The model under review builds one solid part; all positions refer to its coordinate system, in mm. A direction names the side the tool comes from. Round coordinates to 2 decimals unless told otherwise and drop trailing zeros. Loops run counter-clockwise (first coordinate to the right, second up) from the corner with the lowest first, then second, coordinate; pieces in that order, holes last. Notation, with made-up numbers: (8, -32) -> (65, -32) arc R24 ccw to (65, -20) -> close; hole circle Ø9 at (-5.75, -0.75). An arc over 180 degrees is marked (long way). Use a Markdown table: item, result. Add a question column.
1) Consider section C-C on z = 8. Give the boundary of the cut face in (x, y), plus the area to 3 significant figures.
2) Mouldability with a two-part tool opening along X and no side actions: class faces 1 (the cylindrical face through (2.285, 3.584, 14.521)), 2 (the flat face through (13.192, 4.676, 7.888)), 3 (the cylindrical face through (2.285, 3.584, 1.521)), 4 (the flat face through (6, 0, 16)) as released by +X, released by -X, zero draft, split by the parting line, or undercut.
3) For faces 5 (the flat face through (18, 2, 6)), 6 (the flat face through (5, 0, 3)), list the 3-axis set-ups (+Z, -Z, +X, -X, +Y, -Y) from which the entire face can be reached by the end or side of a thin tool; tool diameter is ignored.
4) Consider section D-D on x = 7.5. Give the boundary of the cut face in (y, z).
5) Insertion check: pin 1 (5 mm diameter, centred on x = 2, z = 12, fed in from -Y); pin 2 (1 mm diameter, centred on x = 12, z = 9.5, fed in from +Y); pin 3 (3 mm diameter, centred on x = 14.5, z = 2, fed in from +Y); pin 4 (1.5 mm diameter, centred on x = -3.5, z = 14, fed in from -Y). Each pin has a flat end and moves straight along its axis. Give the tip position at first contact, or say it passes through.
6) Consider section A-A on y = 0. Give the boundary of the cut face in (x, z).
7) Wall thickness on probe 1 along Z at (x, y) = (-4, 4); probe 2 along Y at (x, z) = (0, 13.95); probe 3 along Z at (x, y) = (16.25, 0): over which ranges is each line inside the solid? List them lowest first.
Autodesk Inventor part; units mm, degrees
ref_plane "Work Plane1" through (0, 6.5, 0) normal (0, 1, 0) x (-1, 0, 0)
ref_plane "YZ Plane" through (0, 0, 0) normal (1, 0, 0) x (0, 1, 0)
ref_plane "XY Plane" through (0, 0, 0) normal (0, 0, 1) x (1, 0, 0)
sketch "Sketch1" plane through (0, 0, 0) normal (0, 0, 1) x (1, 0, 0)
  arc A0 (0.2442, 6.4954) -> (0.2442, -6.4954) centre (0, 0) ccw
  line L0 (18, 4) -> (18, -4)
  line L1 (18, 4) -> (0.2442, 6.4954)
  line L2 (0.2442, -6.4954) -> (18, -4)
  point P0 (18, 0)
  dimension "d0" = 13
  dimension "d1" = 8
  dimension "d2" = 18
  dimension "d3" = 82
  dimension "d4" = 82
extrude "Extrusion1" add sketch "Sketch1" along normal blind 16
sketch "Sketch2" plane through (0, 0, 16) normal (0, 0, 1) x (1, 0, 0)
  arc A0 (0.2442, 6.4954) -> (0.2442, -6.4954) centre (0, 0) ccw
  circle A1 centre (0, 0) radius 4.25
  dimension "d7" = 8.5
extrude "Extrusion2" cut sketch "Sketch2" against normal through all
ref_plane "Work Plane1" through (0, 6.5, 0) normal (0, 1, 0) x (-1, 0, 0)
sketch "Sketch3" plane through (0, 6.5, 0) normal (0, 1, 0) x (-1, 0, 0)
  line L0 (6.5, 0) -> (6.5, 16)
  line L1 (6.5, 13) -> (-12, 13)
  line L2 (-12, 13) -> (-12, 3)
  line L3 (-12, 3) -> (6.5, 3)
  line L4 (6.5, 3) -> (6.5, 13)
  line L5 (-18, 0) -> (-18, 16)
  line L6 (6.5, 0) -> (-0.2442, 0)
  line L7 (6.5, 16) -> (-0.2442, 16)
  point P0 (0, 0)
  point P1 (6.5, 3)
  dimension "d11" = 6
  dimension "d12" = 3
  dimension "d13" = 3
extrude "Extrusion3" cut sketch "Sketch3" against normal through all
sketch "Sketch4" plane through (12, -4.8432, 3) normal (-1, 0, 0) x (0, 0, 1)
  line L0 (10, 9.6865) -> (10, 0)
  circle A0 centre (5, 4.8432) radius 2.5
  line L1 (-3, 8.8432) -> (13, 8.8432)
  point P0 (-3, 4.8432)
  dimension "d16" = 5
  dimension "d17" = 4
  dimension "d18" = 5
hole "Hole1" at (12, 0, 8) direction (1, 0, 0) diameter 4.917 depth 6
properties part number "16C - Con Head Crosshead" material "Steel AISI 1020 107 HR"
Result set:
| question | item | result |
|---|---|---|
| 1 | outline | (12, -4.84) -> (18, -4) -> (18, -2.46) -> (12, -2.46) -> close; (12, 2.46) -> (18, 2.46) -> (18, 4) -> (12, 4.84) -> close |
| 1 | area | 23.6 mm2 |
| 2 | face 1 | undercut |
| 2 | face 2 | released by +X |
| 2 | face 3 | undercut |
| 2 | face 4 | zero draft |
| 3 | face 5 | +Z, -Z, +X, +Y, -Y |
| 3 | face 6 | -X, +Y, -Y |
| 4 | outline | (-5.48, 0) -> (5.48, 0) -> (5.48, 3) -> (-5.48, 3) -> close; (-5.48, 13) -> (5.48, 13) -> (5.48, 16) -> (-5.48, 16) -> close |
| 5 | pin 1 | y = -6.5 |
| 5 | pin 2 | y = 4.84 |
| 5 | pin 3 | y = 4.7 |
| 5 | pin 4 | y = -5.89 |
| 6 | outline | (-6.5, 0) -> (-4.25, 0) -> (-4.25, 3) -> (-6.5, 3) -> close; (-6.5, 13) -> (-4.25, 13) -> (-4.25, 16) -> (-6.5, 16) -> close; (4.25, 0) -> (18, 0) -> (18, 5.54) -> (12, 5.54) -> (12, 3) -> (4.25, 3) -> close; (4.25, 13) -> (12, 13) -> (12, 10.46) -> (18, 10.46) -> (18, 16) -> (4.25, 16) -> close |
| 7 | probe 1 | 0 to 3, 13 to 16 |
| 7 | probe 2 | -6.5 to -4.25, 4.25 to 6.5 |
| 7 | probe 3 | 0 to 5.54, 10.46 to 16 |
